from build123d import *

# Parameters (mm, degrees)
SKETCH1_R           = 4.4
BOSS_EXTRUDE1_DEPTH = 2
SKETCH2_R           = 2.4
BOSS_EXTRUDE2_DEPTH = 2
SKETCH3_W           = 3
SKETCH3_H           = 3
BOSS_EXTRUDE3_DEPTH = 5


with BuildPart() as part:
    # Sketch1 → Boss-Extrude1 (new body)
    with BuildSketch(Plane(origin=(0, 0, 0), x_dir=(1, 0, 0), z_dir=(0, 1, 0))):
        with Locations(Location((0, 0, 0), (0, 0, 270))):
            Circle(SKETCH1_R)
    extrude(amount=BOSS_EXTRUDE1_DEPTH)

    # Sketch2 → Boss-Extrude2 (add)
    with BuildSketch(Plane(origin=(0, 2, 0), x_dir=(1, 0, 0), z_dir=(0, 1, 0))):
        with Locations(Location((0, 0, 0), (0, 0, 270))):
            Circle(SKETCH2_R)
    extrude(amount=BOSS_EXTRUDE2_DEPTH)

    # Sketch3 → Boss-Extrude3 (add)
    with BuildSketch(Plane(origin=(0, 4, 0), x_dir=(1, 0, 0), z_dir=(0, 1, 0))):
        with BuildLine():
            ThreePointArc((1.5, 1.8734994), (0, 2.4), (-1.5, 1.8734994))
            Line((-1.5, 1.8734994), (-1.5, 1.5))
            Line((-1.5, 1.5), (1.5, 1.5))
            Line((1.5, 1.5), (1.5, 1.8734994))
        make_face()
        Rectangle(SKETCH3_W, SKETCH3_H)
        with BuildLine():
            Line((1.5, -1.5), (-1.5, -1.5))
            Line((-1.5, -1.5), (-1.5, -1.8734994))
            ThreePointArc((-1.5, -1.8734994), (0, -2.4), (1.5, -1.8734994))
            Line((1.5, -1.8734994), (1.5, -1.5))
        make_face()
    extrude(amount=BOSS_EXTRUDE3_DEPTH)


solid = part.part
For this review, take the finished solid that the model builds, in its own axes (mm). A direction names the side the tool comes from. Round coordinates to 2 decimals unless told otherwise and drop trailing zeros. Loops run counter-clockwise (first coordinate to the right, second up) from the corner with the lowest first, then second, coordinate; pieces in that order, holes last. Notation, with made-up numbers: (9, 49.5) - (30, 49.5) arc R28 cw to (30, 67.5) - close; hole circle Ø2 at (22, -2). An arc over 180 degrees is marked (long way). Put each result on its own line as item: value. Start each with the question number.
1. Consider section A-A on z = 0. State the section outline as (x, y) points, plus the area to 3 significant figures.
2. Consider section B-B on y = 5. State the section outline as (x, z) points.
3. Insertion check: P1, Ø1, axis at x = -3.5, y = 1.5, coming from the +Z side; P2, Ø1, axis at y = 8, z = 0.5, coming from the +X side; P3, Ø2, axis at x = -0.5, y = 5, coming from the -Z side. Each pin has a flat end and moves straight along its axis. Give the tip position at first contact, or say it passes through.
4. Consider section D-D on z = 1.5. State the section outline as (x, y) points, plus the area to 3 significant figures.
5. For probe 1 along Y at (x, z) = (-1.5, 2.75); probe 2 along X at (y, z) = (7, 1); probe 3 along Z at (x, y) = (-2.75, 1.5), list the stretches that pass through material, from the lowest coordinate up. Write a range as [from, to].
6. For faces 1 (the cylindrical face through (4.363, 0.986, -0.573)), 2 (the flat face through (0, 0, 0)), 3 (the flat face through (2, 4, 0)), 4 (the flat face through (-2, 2, 2)), 5 (the flat face through (-1.5, 6, 0)), list the 3-axis set-ups (+Z, -Z, +X, -X, +Y, -Y) from which the entire face can be reached by the end or side of a thin tool; tool diameter is ignored.
7. Consider section C-C on x = -2.25. State the section outline as (y, z) points.
Result sheet:
1. outline: (-4.4, 0) - (4.4, 0) - (4.4, 2) - (2.4, 2) - (2.4, 4) - (1.5, 4) - (1.5, 9) - (-1.5, 9) - (-1.5, 4) - (-2.4, 4) - (-2.4, 2) - (-4.4, 2) - close
1. area: 42.2 mm^2
2. outline: (-1.5, -1.87) arc R2.4 ccw to (1.5, -1.87) - (1.5, 1.87) arc R2.4 ccw to (-1.5, 1.87) - close
3. P1: z = 3.22
3. P2: x = 1.5
3. P3: z = -2.4
4. outline: (-4.14, 0) - (4.14, 0) - (4.14, 2) - (1.87, 2) - (1.87, 4) - (1.5, 4) - (1.5, 9) - (-1.5, 9) - (-1.5, 4) - (-1.87, 4) - (-1.87, 2) - (-4.14, 2) - close
4. area: 39.0 mm^2
5. probe 1: [0, 2]
5. probe 2: [-1.5, 1.5]
5. probe 3: [-3.43, 3.43]
6. face 1: +Y, -Y
6. face 2: +Z, -Z, +X, -X, -Y
6. face 3: +Z, -Z, +X, +Y
6. face 4: +Y
6. face 5: +Z, -Z, -X, +Y
7. outline: (0, -3.78) - (2, -3.78) - (2, -0.84) - (4, -0.84) - (4, 0.84) - (2, 0.84) - (2, 3.78) - (0, 3.78) - close
